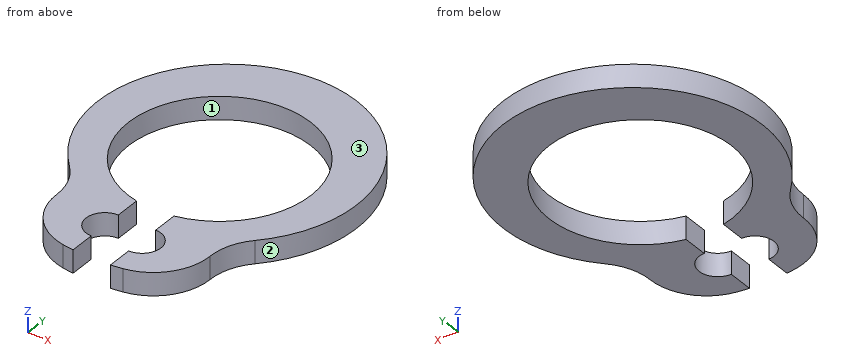
Autodesk Inventor part; units mm, degrees
ref_plane "Work Plane1" through (0, -3, 0) normal (-1, 0, 0) x (0, 0, 1)
ref_plane "YZ Plane" through (0, 0, 0) normal (1, 0, 0) x (0, 1, 0)
ref_plane "XZ Plane" through (0, 0, 0) normal (0, 1, 0) x (-1, 0, 0)
sketch "Эскиз1" plane through (0, 0, 0) normal (0, 0, 1) x (1, 0, 0)
  line L0 (-6, 0) -> (6, 0) construction
  arc A0 (0.575, -5.7403) -> (-0.575, -5.7403) centre (0, -3) ccw
  line L1 (0, 4.8751) -> (0, -17.3507)
  line L2 (-8.435, 0) -> (8.435, 0)
  arc A1 (-0.575, -6.5153) -> (-0.575, -7.6653) centre (-0.575, -7.0903) ccw
  line L3 (-0.575, -5.7403) -> (-0.575, -6.5153)
  line L4 (-0.575, -7.6653) -> (-0.575, -8.4403)
  line L5 (-0.575, -6.5402) -> (-0.575, -13.29) construction
  line L6 (-2.7947, 1.3) -> (3.6722, 1.3) construction
  circle A2 centre (-0.575, -7.0903) radius 1.725 construction
  line L7 (0, -3) -> (-6.3375, -12.8769) construction
  arc A3 (2.8464, -5.4497) -> (-2.8464, -5.4497) centre (0, -2.675) ccw
  arc A4 (-0.9228, -8.3922) -> (-0.575, -8.4403) centre (0, -3) ccw
  arc A5 (-2.3567, -6.6729) -> (-0.9228, -8.3922) centre (-0.6318, -6.692) ccw
  arc A6 (-2.3567, -6.6729) -> (-2.8464, -5.4497) centre (-4.0816, -6.6538) ccw
  arc A7 (0.575, -7.6653) -> (0.575, -6.5153) centre (0.575, -7.0903) ccw
  line L8 (0.575, -5.7403) -> (0.575, -6.5153)
  line L9 (0.575, -7.6653) -> (0.575, -8.4403)
  line L10 (0.575, -6.5402) -> (0.575, -13.29) construction
  arc A8 (0.575, -8.4403) -> (0.9228, -8.3922) centre (0, -3) ccw
  arc A9 (0.9228, -8.3922) -> (2.3567, -6.6729) centre (0.6318, -6.692) ccw
  arc A10 (2.8464, -5.4497) -> (2.3567, -6.6729) centre (4.0816, -6.6538) ccw
  dimension "d1" = 6
  dimension "d0" = 5.6
  dimension "d2" = 2.7
  dimension "d3" = 0.575
  dimension "d8" = 0.575
  dimension "d9" = 1.35
  dimension "d10" = 1.3
  dimension "d11" = 3.45
  dimension "d12" = 0.325
  dimension "d13" = 1.725
  dimension "d14" = 1.725
extrude "Базовый элемент" add sketch "Эскиз1" along normal blind 0.7
ref_plane "Work Plane1" through (0, -3, 0) normal (-1, 0, 0) x (0, 0, 1)
equation "\"d1\" = WD"
equation "\"d0\" = ND"
equation "\"d2\" = SRB2"
equation "\"d3\" = 0.5 * SD5"
equation "\"d8\" = 0.5 * SD5"
equation "\"d9\" = 0.5 * SRB2"
equation "\"d10\" = SRB1"
equation "\"d11\" = 3 * SD5"
equation "\"d12\" = 0.25 * SRB1"
equation "\"d13\" = 1.5 * SD5"
equation "\"d14\" = 1.5 * SD5"
equation "\"d4\" = SD"
equation "\"WD\" = WDMIN"
equation "\"SD\" = 0.7"
equation "\"SRB1\" = 1.3"
equation "\"ND\" = 5.6"
equation "\"SRB2\" = 2.7"
equation "\"SD5\" = 1.15"
equation "\"WDMIN\" = 6"
equation "\"SD3\" = 5.4"
equation "\"WDMAX\" = 7"
equation "\"SNB\" = 0.8"
equation "\"BUBRMI\" = 0.6"
properties part number "Кольцо C6 ГОСТ 13942-86" material "Сталь, мягкая"
Can you work these out from the model? Positions are in its coordinate system, mm. Face numbers are marked on the shaded views. Round coordinates to 2 decimals unless told otherwise and drop trailing zeros. Loops run counter-clockwise (first coordinate to the right, second up) from the corner with the lowest first, then second, coordinate; pieces in that order, holes last. Notation, with made-up numbers: M 6,88.5 L 35,88.5 A10 ccw 35,107.5 Z; hole C 66.5,2.5 d5. An arc over 180 degrees is marked long. Write item = value, one per line. Start each with the question number.
(1) Suppose I cut it at C-C on y = -0.5. Write out the boundary of the cut face in (x, z), plus the area to 3 significant figures.
(2) Suppose I cut it at B-B on x = 0. Write out the boundary of the cut face in (y, z).
(3) Suppose I cut it at D-D on z = 0.45. Write out the boundary of the cut face in (x, y) (3 decimals), plus the area to 3 significant figures.
(4) If we mould it in two halves opening along X, with no side actions, what happens to the marked faces 1, 2 and 3? For each: released by +X, released by -X, zero draft, split by the parting line, or undercut.
(5) Suppose I cut it at A-A on y = -3. Write out the boundary of the cut face in (x, z), plus the area to 3 significant figures.
(6) I need wall thicknesses on line 1 along Y through (x, z) = (0, 0.4); line 2 along X through (y, z) = (-3, 0.55); line 3 along Y through (x, z) = (1.5, 0.5). Which ranges of each line are inside material? Lowest first, please.
Answer block:
q1.outline = M -3.33,0 L -1.26,0 L -1.26,0.7 L -3.33,0.7 Z; M 1.26,0 L 3.33,0 L 3.33,0.7 L 1.26,0.7 Z
q1.area = 2.89 mm²
q2.outline = M -0.2,0 L 1.3,0 L 1.3,0.7 L -0.2,0.7 Z
q3.outline = M -2.846,-5.45 A1.725 cw -2.357,-6.673 A1.725 ccw -0.923,-8.392 A5.48 ccw -0.575,-8.44 L -0.575,-7.665 A0.575 cw -0.575,-6.515 L -0.575,-5.74 A2.8 cw long 0.575,-5.74 L 0.575,-6.515 A0.575 cw 0.575,-7.665 L 0.575,-8.44 A5.461 ccw 0.923,-8.392 A1.725 ccw 2.357,-6.673 A1.725 cw 2.846,-5.45 A3.975 ccw long Z
q3.area = 29.3 mm²
q4.face_1 = undercut
q4.face_2 = split by the parting line
q4.face_3 = zero draft
q5.outline = M -3.96,0 L -2.8,0 L -2.8,0.7 L -3.96,0.7 Z; M 2.8,0 L 3.96,0 L 3.96,0.7 L 2.8,0.7 Z
q5.area = 1.63 mm²
q6.line_1 = -0.2 to 1.3
q6.line_2 = -3.96 to -2.8, 2.8 to 3.96
q6.line_3 = -8.18 to -5.36, -0.64 to 1.01
